Input: part model. Units: mm. Frame: model coordinates. A direction names the side the tool comes from. Coordinates: 2 decimals unless noted, no trailing zeros. Loops run counter-clockwise (first coordinate to the right, second up) from the corner with the lowest first, then second, coordinate; pieces in that order, holes last.
Item 1: Section A-A on y = 3. Return loops of the section in (x, z).
Item 2: Ray query, line 1 along X through (y, z) = (-5.5, 465); line 2 along Y through (x, z) = (4.5, 41.5); line 3 along Y through (x, z) = (6.5, 150). Return the intervals inside material, ascending.
Item 3: Pull-direction query (Y, two-part tool) for faces 1 (the flat face through (7.5, 0, 271)), 2 (the flat face through (-5.5, 0, 271)), 3 (the flat face through (-2, -15, 271)), 4 (the flat face through (2, 15, 271)); classes: released by +Y, released by -Y, zero draft, split by the parting line, or undercut.
Item 4: Reachability of faces 5 (the flat face through (5.5, 0, 271)), 6 (the flat face through (-7, 0, 0)) from +Z, -Z, +X, -X, +Y, -Y: full face, straight path, thin tool, end or side. Return the list, or none.
Item 5: Section B-B on z = 203. Return loops of the section in (x, y), and give its area (3 significant figures).
Autodesk Inventor part; units mm, degrees
ref_plane "YZ Plane" through (0, 0, 0) normal (1, 0, 0) x (0, 1, 0)
ref_plane "XZ Plane" through (0, 0, 0) normal (0, 1, 0) x (-1, 0, 0)
ref_plane "XY Plane" through (0, 0, 0) normal (0, 0, 1) x (1, 0, 0)
sketch "スケッチ1" plane through (0, 0, 0) normal (0, 0, 1) x (1, 0, 0)
  line L0 (7.5, 15) -> (-7.5, 15)
  line L1 (-7.5, 15) -> (-7.5, -15)
  line L2 (-7.5, -15) -> (7.5, -15)
  line L3 (7.5, -15) -> (7.5, 15)
  line L4 (7.5, 15) -> (-7.5, -15) construction
  line L5 (-7.5, 15) -> (7.5, -15) construction
  line L6 (-5.5, 13) -> (5.5, 13)
  line L7 (5.5, 13) -> (5.5, -13)
  line L8 (5.5, -13) -> (-5.5, -13)
  line L9 (-5.5, -13) -> (-5.5, 13)
  point P0 (0, 0)
  dimension "d0" = 15
  dimension "d1" = 30
  dimension "d2" = 2
extrude "押し出し1" add sketch "スケッチ1" along normal blind 549
sketch "スケッチ2" plane through (-7.5, 15, 0) normal (0, 1, 0) x (1, 0, 0)
  circle A0 centre (7.5, -10) radius 1.6
  circle A1 centre (7.5, -25) radius 1.6
  circle A2 centre (7.5, -40) radius 1.6
  line L0 (15, 0) -> (0, 0)
  circle A3 centre (7.5, -255) radius 1.6
  circle A4 centre (7.5, -270) radius 1.6
  circle A5 centre (7.5, -539) radius 1.6
  circle A6 centre (7.5, -524) radius 1.6
  point P0 (7.5, 0)
  point P1 (7.5, 0)
  dimension "d5" = 3.2
  dimension "d6" = 3.2
  dimension "d7" = 3.2
  dimension "d8" = 10
  dimension "d9" = 15
  dimension "d10" = 15
  dimension "d11" = 3.2
  dimension "d12" = 3.2
  dimension "d13" = 215
  dimension "d14" = 15
  dimension "d15" = 3.2
  dimension "d16" = 3.2
  dimension "d17" = 15
  dimension "d18" = 484
extrude "押し出し2" cut sketch "スケッチ2" against normal through all
sketch "スケッチ3" plane through (7.5, -15, 0) normal (1, 0, 0) x (0, 0, -1)
  circle A0 centre (-120, 7.5) radius 1.6
  circle A1 centre (-150, 7.5) radius 1.6
  line L0 (0, 0) -> (-549, 0)
  point P0 (0, 15)
  dimension "d21" = 3.2
  dimension "d22" = 3.2
  dimension "d23" = 30
  dimension "d24" = 7.5
  dimension "d25" = 120
extrude "押し出し3" cut sketch "スケッチ3" against normal through all
properties part number "オムニ_角柱1" material "アルミニウム 6061"
Results found:
1. outline: (-7.5, 0) - (-5.5, 0) - (-5.5, 549) - (-7.5, 549) - close; (5.5, 0) - (7.5, 0) - (7.5, 549) - (5.5, 549) - close
2. line 1: x = -7.5 to -5.5, 5.5 to 7.5
2. line 2: y = -15 to -13, 13 to 15
2. line 3: y = -15 to -9.1, -5.9 to 15
3. face 1: zero draft
3. face 2: undercut
3. face 3: released by -Y
3. face 4: released by +Y
4. face 5: +Z, -Z
4. face 6: -Z, +X, -X, +Y, -Y
5. outline: (-7.5, -15) - (7.5, -15) - (7.5, 15) - (-7.5, 15) - close; hole (-5.5, -13) - (5.5, -13) - (5.5, 13) - (-5.5, 13) - close
5. area: 164 mm2
